Build history of the part. All positions in model axes, mm. Round coordinates to 2 decimals unless told otherwise and drop trailing zeros. Order: outer loops, then holes, each group sorted by start corner. A loop starts at its lowest first (then second) coordinate and runs counter-clockwise, first axis right, second up. Notation, with made-up numbers: M -7.5,22.5 L 17.5,22.5 A20 ccw 17.5,59.5 Z; hole C 54.25,51 d10. An arc over 180 degrees is marked long. Use CSV: the item, a comma, the result in double quotes.
from build123d import *

# Parameters (mm, degrees)
SKETCH1_R           = 3
BOSS_EXTRUDE1_DEPTH = 30
CHAMFER1_SIZE       = 1
CHAMFER1_SIZE2      = 0.363970234
CHAMFER2_SIZE       = 1
CHAMFER2_SIZE2      = 0.363970234


with BuildPart() as part:
    # Sketch1 → Boss-Extrude1 (new body)
    with BuildSketch(Plane(origin=(0, 0, 0), x_dir=(1, 0, 0), z_dir=(0, 1, 0))):
        Circle(SKETCH1_R)
    extrude(amount=BOSS_EXTRUDE1_DEPTH)

    # Chamfer1
    chamfer1_edges = [part.edges().sort_by_distance(p)[0] for p in [
        (-3, 30, 0),
    ]]
    chamfer1_side = [part.faces().sort_by_distance(p)[0] for p in [
        (-3, 15, 0),
    ]]
    chamfer(chamfer1_edges, length=CHAMFER1_SIZE, length2=CHAMFER1_SIZE2, reference=chamfer1_side[0])

    # Chamfer2
    chamfer2_edges = [part.edges().sort_by_distance(p)[0] for p in [
        (-3, 0, 0),
    ]]
    chamfer2_side = [part.faces().sort_by_distance(p)[0] for p in [
        (-3, 14.5, 0),
    ]]
    chamfer(chamfer2_edges, length=CHAMFER2_SIZE, length2=CHAMFER2_SIZE2, reference=chamfer2_side[0])


solid = part.part
(1) Wall check: line 1 (Z direction, x = 0.2, y = 3.25); line 2 (X direction, y = 25.5, z = -0.75); line 3 (Z direction, x = 1.3, y = 22.5). Give the ranges that are in metal, low to high. Write a range as from..to.
Answer block:
line 1,"z = -2.99..2.99"
line 2,"x = -2.9..2.9"
line 3,"z = -2.7..2.7"
(2) Drop a flat-ended pin along its axis: pin 1 (1 mm diameter, centred on y = 24, z = -2.5, fed in from +X). Give the stop position or say it passes through.
Answer block:
pin 1,"stops at x = 2.24"
(3) Cut at A-A, the plane y = 27.5. Give the cut face in (x, z).
Answer block:
outline,"C 0,0 d6"
